Geometry check sheet. Reference: the model listing, model coordinates, mm. A direction names the side the tool comes from. Give positions to 0.01 mm unless a question says otherwise; leave off trailing zeros. Loops run counter-clockwise (first coordinate to the right, second up) from the corner with the lowest first, then second, coordinate; pieces in that order, holes last. Notation, with made-up numbers: (-11.5, -33) - (-3.5, -33) arc R31 cw to (-3.5, 4) - close; hole circle Ø1 at (31.25, 40). An arc over 180 degrees is marked (long way). Use a Markdown table: item, result. Add a question column.
1. Cross-section at C-C on y = -21.5. Enter the section's corners in (x, z).
2. Cross-section at B-B on z = 729.5. Enter the section's corners in (x, y), and give its area (3 significant figures).
3. Set-up check for faces 4 (the flat face through (25.4, -1, 451)), 5 (the flat face through (0, -1, 812.8)), 6 (the flat face through (0, 0, 50)): record each of +Z, -Z, +X, -X, +Y, -Y from which the full face is reachable in a straight line by a thin tool's end or side.
4. Depth check by flat-ended pin: P1, Ø15, axis at x = 0, z = 863, coming from the +Y side. Enter the tip coordinate at first touch or a pass-through.
5. Draft check along X on faces 1 (the flat face through (-25.4, -1, 451)), 2 (the flat face through (0, 25, 838.2)), 3 (the flat face through (-12.7, -1, 763)). Enter one of: pulls with the +X half, pulls with the -X half, needs draft (parallel to the pull), parting line crosses it, or undercut.
6. Material ranges on L1, parallel to Z at x = 22, y = 39.5; L2, parallel to Z at x = 10, y = 3.5; L3, parallel to X at y = -39, z = 722, recorded low to high.
7. Cross-section at A-A on y = 23.5. Enter the section's corners in (x, z), and give its area (3 significant figures).
from build123d import *

# Parameters (mm, degrees)
SKETCH1_W           = 50.8
SKETCH1_H           = 101.6
BOSS_EXTRUDE1_DEPTH = 914.4
SKETCH2_W           = 50.8
SKETCH2_H           = 50.8
CUT_EXTRUDE1_DEPTH  = 918.217880332
SKETCH3_W           = 25.4
SKETCH3_H           = 101.6
CUT_EXTRUDE2_DEPTH  = 921.377683345


with BuildPart() as part:
    # Sketch1 → Boss-Extrude1 (new body)
    with BuildSketch(Plane.XY):
        Rectangle(SKETCH1_W, SKETCH1_H)
    extrude(amount=BOSS_EXTRUDE1_DEPTH)

    # Sketch2 → Cut-Extrude1 (cut, symmetric)
    with BuildSketch(Plane(origin=(25.4, 0, 0), x_dir=(0, 0, -1), z_dir=(1, 0, 0))):
        with Locations((304.8, 25.4)):
            Rectangle(SKETCH2_W, SKETCH2_H)
        with Locations((-863.6, 25.4)):
            Rectangle(SKETCH2_W, SKETCH2_H)
        with Locations((1473.2, 25.4)):
            Rectangle(SKETCH2_W, SKETCH2_H)
    cut_extrude1 = extrude(amount=CUT_EXTRUDE1_DEPTH, both=True, mode=Mode.SUBTRACT)

    # Mirror1: Cut-Extrude1 across plane
    add(cut_extrude1.mirror(Plane.XY.offset(457.2)), mode=Mode.SUBTRACT)

    # Sketch3 → Cut-Extrude2 (cut, through all)
    with BuildSketch(Plane(origin=(0, -50.8, 0), x_dir=(-1, 0, 0), z_dir=(0, -1, 0))):
        with Locations((0, -762)):
            Rectangle(SKETCH3_W, SKETCH3_H)
    extrude(amount=-CUT_EXTRUDE2_DEPTH, mode=Mode.SUBTRACT)


solid = part.part
Values found:
| question | item | result |
|---|---|---|
| 1 | outline | (-25.4, 0) - (25.4, 0) - (25.4, 914.4) - (-25.4, 914.4) - close; hole (-12.7, 711.2) - (12.7, 711.2) - (12.7, 812.8) - (-12.7, 812.8) - close |
| 2 | outline | (-25.4, -50.8) - (-12.7, -50.8) - (-12.7, 50.8) - (-25.4, 50.8) - close; (12.7, -50.8) - (25.4, -50.8) - (25.4, 50.8) - (12.7, 50.8) - close |
| 2 | area | 2,580 mm2 |
| 3 | face 4 | +Z, -Z, +X, +Y, -Y |
| 3 | face 5 | +Y, -Y |
| 3 | face 6 | +X, -X, +Y |
| 4 | P1 | stops at y = 0 |
| 5 | face 1 | pulls with the -X half |
| 5 | face 2 | needs draft |
| 5 | face 3 | undercut |
| 6 | L1 | z = 0 to 25.4, 76.2 to 838.2, 889 to 914.4 |
| 6 | L2 | z = 0 to 25.4, 76.2 to 711.2, 812.8 to 838.2, 889 to 914.4 |
| 6 | L3 | x = -25.4 to -12.7, 12.7 to 25.4 |
| 7 | outline | (-25.4, 0) - (25.4, 0) - (25.4, 25.4) - (-25.4, 25.4) - close; (-25.4, 76.2) - (25.4, 76.2) - (25.4, 838.2) - (-25.4, 838.2) - close; (-25.4, 889) - (25.4, 889) - (25.4, 914.4) - (-25.4, 914.4) - close; hole (-12.7, 711.2) - (12.7, 711.2) - (12.7, 812.8) - (-12.7, 812.8) - close |
| 7 | area | 38,700 mm2 |
